Geometry check sheet. Reference: the model listing, model coordinates, mm. Face numbers are marked on the shaded views. A direction names the side the tool comes from. Give positions to 0.01 mm unless a question says otherwise; leave off trailing zeros. Write each loop counter-clockwise with the first axis right and the second up, starting at its lowest first coordinate (ties: lowest second). Pieces come first, ordered by that corner, then holes.
(1) Thickness scan on line 1 along Z through (x, y) = (-20, 0.6); line 2 along X through (y, z) = (13.5, -7.5); line 3 along Z through (x, y) = (-38, 1.6). Record the ranges inside material, lowest first.
(2) Cross-section at A-A (x = -31). Record the boundary of the cut face in (y, z).
(3) Depth check by flat-ended pin: P1, Ø13.5, axis at x = 20, z = 0, coming from the +Y side; P2, Ø0.8, axis at x = 20.5, z = 14.5, coming from the +Y side. Enter the tip coordinate at first touch or a pass-through.
(4) Cross-section at D-D (y = 4). Record the boundary of the cut face in (x, z).
(5) Tool access check on the marked faces 5 and 6. Record the directions out of +Z, -Z, +X, -X, +Y, -Y that give a thin tool (end or side, any length) a straight path to the whole face; none if there is none.
(6) Cross-section at B-B (y = 15.5). Record the boundary of the cut face in (x, z), and give its area (3 significant figures).
(7) Mould release check, pull along Z, two halves, no side actions. Record for the marked faces 1, 2, 3 and 4: +Z half, -Z half, draft (parallel to the pull), parting line (faces both ways), or undercut.
(8) Cross-section at C-C (x = 20). Record the boundary of the cut face in (y, z).
```python
from build123d import *

# Parameters (mm, degrees)
SKETCH2_W              = 105
SKETCH2_H              = 32
BOSS_EXTRUDE1_DEPTH    = 40
SKETCH3_W              = 100
SKETCH3_H              = 32
CUT_EXTRUDE1_DEPTH     = 30
SKETCH4_W              = 100
SKETCH4_H              = 27
CUT_EXTRUDE2_DEPTH     = 7.5
F_10_0MM_DOWEL_HOLE1_D = 10.2
F_2_5MM_DOWEL_HOLE1_D  = 2.6
CIRPATTERN1_COUNT      = 8
F_2_5MM_DOWEL_HOLE2_D  = 2.6
LPATTERN1_COUNT        = 3
LPATTERN1_PITCH        = 38
MIRROR1_COPY_1_D       = 2.6
MIRROR1_COPY_2_D       = 2.6
MIRROR1_COPY_3_D       = 2.6
MIRROR1_COPY_4_D       = 2.6
MIRROR1_COPY_5_D       = 2.6
MIRROR1_COPY_6_D       = 2.6
MIRROR1_COPY_7_D       = 2.6
CUT_EXTRUDE3_DEPTH     = 72.75
F_2_5MM_DOWEL_HOLE3_D  = 2.6
CIRPATTERN3_COUNT      = 5
CIRPATTERN3_ANGLE      = 180
SKETCH18_W             = 16
SKETCH18_H             = 4
CUT_EXTRUDE4_DEPTH     = 72.75
SKETCH19_W             = 10
SKETCH19_H             = 10
SKETCH19_W_2           = 4.5
CUT_EXTRUDE5_DEPTH     = 145.5


with BuildPart() as part:
    # Sketch2 → Boss-Extrude1 (new body)
    with BuildSketch(Plane(origin=(0, 0, 0), x_dir=(1, 0, 0), z_dir=(0, 1, 0))):
        Rectangle(SKETCH2_W, SKETCH2_H)
    extrude(amount=BOSS_EXTRUDE1_DEPTH)

    # Sketch3 → Cut-Extrude1 (cut)
    with BuildSketch(Plane(origin=(0, 40, 0), x_dir=(1, 0, 0), z_dir=(0, 1, 0))):
        Rectangle(SKETCH3_W, SKETCH3_H)
    extrude(amount=-CUT_EXTRUDE1_DEPTH, mode=Mode.SUBTRACT)

    # Sketch4 → Cut-Extrude2 (cut)
    with BuildSketch(Plane(origin=(0, 10, 0), x_dir=(1, 0, 0), z_dir=(0, 1, 0))):
        Rectangle(SKETCH4_W, SKETCH4_H)
    extrude(amount=-CUT_EXTRUDE2_DEPTH, mode=Mode.SUBTRACT)

    # 10.0mm Dowel Hole1 (through all)
    with Locations(Plane(origin=(0, 0, 0), x_dir=(-1, 0, 0), z_dir=(0, -1, 0))):
        with Locations((-20, 0), (20, 0)):
            Hole(F_10_0MM_DOWEL_HOLE1_D / 2)

    # 2.5mm Dowel Hole1 (through all)
    with Locations(Plane(origin=(0, 0, 0), x_dir=(-1, 0, 0), z_dir=(0, -1, 0))):
        with Locations((-20, 11)):
            f_2_5mm_dowel_hole1 = Hole(F_2_5MM_DOWEL_HOLE1_D / 2)

    # CirPattern1: 2.5mm Dowel Hole1 ×8 about axis
    cirpattern1_axis = Axis((20, 0, 0), (0, 1, 0))
    for i in range(1, CIRPATTERN1_COUNT):
        add(f_2_5mm_dowel_hole1.rotate(cirpattern1_axis, i * 360 / CIRPATTERN1_COUNT), mode=Mode.SUBTRACT)

    # 2.5mm Dowel Hole2 (through all)
    with Locations(Plane(origin=(0, 0, 0), x_dir=(-1, 0, 0), z_dir=(0, -1, 0))):
        with Locations((-38, 11), (-38, -11)):
            f_2_5mm_dowel_hole2 = Hole(F_2_5MM_DOWEL_HOLE2_D / 2)

    # LPattern1: 2.5mm Dowel Hole2 ×3
    with Locations(*[(-i * LPATTERN1_PITCH, 0, 0) for i in range(1, LPATTERN1_COUNT)]):
        add(f_2_5mm_dowel_hole2, mode=Mode.SUBTRACT)

    # Mirror1: 2.5mm Dowel Hole1 across plane
    add(f_2_5mm_dowel_hole1.mirror(Plane(origin=(0, 0, 0), x_dir=(0, 0, 1), z_dir=(1, 0, 0))), mode=Mode.SUBTRACT)

    # Mirror1 copy 1 (through all)
    with Locations(Plane(origin=(-5.857864376, 0, 14.142135624), x_dir=(0.707106781, 0, 0.707106781), z_dir=(0, -1, 0))):
        with Locations((-20, -11)):
            Hole(MIRROR1_COPY_1_D / 2)

    # Mirror1 copy 2 (through all)
    with Locations(Plane(origin=(-20, 0, 20), x_dir=(0, 0, 1), z_dir=(0, -1, 0))):
        with Locations((-20, -11)):
            Hole(MIRROR1_COPY_2_D / 2)

    # Mirror1 copy 3 (through all)
    with Locations(Plane(origin=(-34.142135624, 0, 14.142135624), x_dir=(-0.707106781, 0, 0.707106781), z_dir=(0, -1, 0))):
        with Locations((-20, -11)):
            Hole(MIRROR1_COPY_3_D / 2)

    # Mirror1 copy 4 (through all)
    with Locations(Plane(origin=(-40, 0, 0), x_dir=(-1, 0, 0), z_dir=(0, -1, 0))):
        with Locations((-20, -11)):
            Hole(MIRROR1_COPY_4_D / 2)

    # Mirror1 copy 5 (through all)
    with Locations(Plane(origin=(-34.142135624, 0, -14.142135624), x_dir=(-0.707106781, 0, -0.707106781), z_dir=(0, -1, 0))):
        with Locations((-20, -11)):
            Hole(MIRROR1_COPY_5_D / 2)

    # Mirror1 copy 6 (through all)
    with Locations(Plane(origin=(-20, 0, -20), x_dir=(0, 0, -1), z_dir=(0, -1, 0))):
        with Locations((-20, -11)):
            Hole(MIRROR1_COPY_6_D / 2)

    # Mirror1 copy 7 (through all)
    with Locations(Plane(origin=(-5.857864376, 0, -14.142135624), x_dir=(0.707106781, 0, -0.707106781), z_dir=(0, -1, 0))):
        with Locations((-20, -11)):
            Hole(MIRROR1_COPY_7_D / 2)

    # Sketch14 → Cut-Extrude3 (cut, symmetric)
    with BuildSketch(Plane(origin=(0, 0, 0), x_dir=(0, 0, -1), z_dir=(1, 0, 0))):
        with BuildLine():
            Line((-5.1, 40), (5.1, 40))
            Line((5.1, 40), (5.1, 37))
            ThreePointArc((5.1, 37), (0, 31.9), (-5.1, 37))
            Line((-5.1, 37), (-5.1, 40))
        make_face()
    extrude(amount=CUT_EXTRUDE3_DEPTH, both=True, mode=Mode.SUBTRACT)

    # 2.5mm Dowel Hole3 (through all)
    with Locations(Plane(origin=(52.5, 0, 0), x_dir=(0, 0, -1), z_dir=(1, 0, 0))):
        with Locations((11, 37)):
            f_2_5mm_dowel_hole3 = Hole(F_2_5MM_DOWEL_HOLE3_D / 2)

    # CirPattern3: 2.5mm Dowel Hole3 ×5 about axis
    cirpattern3_axis = Axis((0, 37, 0), (-1, 0, 0))
    for i in range(1, CIRPATTERN3_COUNT):
        add(f_2_5mm_dowel_hole3.rotate(cirpattern3_axis, i * CIRPATTERN3_ANGLE / (CIRPATTERN3_COUNT - 1)), mode=Mode.SUBTRACT)

    # Sketch18 → Cut-Extrude4 (cut, symmetric)
    with BuildSketch(Plane(origin=(0, 0, 0), x_dir=(0, 0, -1), z_dir=(1, 0, 0))):
        with Locations((0, 16.5)):
            Rectangle(SKETCH18_W, SKETCH18_H)
        with Locations((0, 8.5)):
            Rectangle(SKETCH18_W, SKETCH18_H)
    extrude(amount=CUT_EXTRUDE4_DEPTH, both=True, mode=Mode.SUBTRACT)

    # Sketch19 → Cut-Extrude5 (cut)
    with BuildSketch(Plane.XZ):
        Rectangle(SKETCH19_W, SKETCH19_H)
        with Locations((40.5, 0)):
            Rectangle(SKETCH19_W_2, SKETCH19_H)
        with Locations((-40.5, 0)):
            Rectangle(SKETCH19_W_2, SKETCH19_H)
    extrude(amount=-CUT_EXTRUDE5_DEPTH, mode=Mode.SUBTRACT)


solid = part.part
```
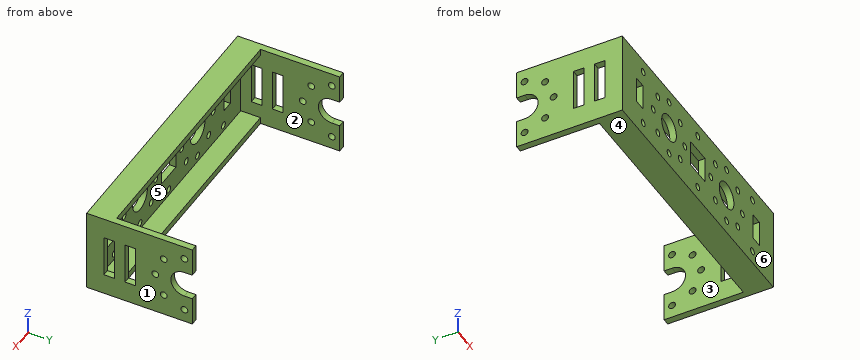
Reply:
1. line 1: z = -16 to -12.3, -9.7 to -5.1, 5.1 to 9.7, 12.3 to 16
1. line 2: x = -52.5 to -50, 50 to 52.5
1. line 3: z = -16 to -12.3, -9.7 to 9.7, 12.3 to 16
2. outline: (0, -16) - (10, -16) - (10, -13.5) - (2.5, -13.5) - (2.5, -1.3) - (0, -1.3) - close; (0, 1.3) - (2.5, 1.3) - (2.5, 13.5) - (10, 13.5) - (10, 16) - (0, 16) - close
3. P1: stops at y = 2.5
3. P2: stops at y = 10
4. outline: (-52.5, -16) - (52.5, -16) - (52.5, 16) - (-52.5, 16) - close; hole (-50, -13.5) - (50, -13.5) - (50, 13.5) - (-50, 13.5) - close
5. face 5: +Y
5. face 6: +Z, -Z, +X, -X, -Y
6. outline: (-52.5, -16) - (-50, -16) - (-50, -8) - (-52.5, -8) - close; (-52.5, 8) - (-50, 8) - (-50, 16) - (-52.5, 16) - close; (50, -16) - (52.5, -16) - (52.5, -8) - (50, -8) - close; (50, 8) - (52.5, 8) - (52.5, 16) - (50, 16) - close
6. area: 80.0 mm2
7. face 1: draft
7. face 2: undercut
7. face 3: undercut
7. face 4: -Z half
8. outline: (0, -16) - (10, -16) - (10, -13.5) - (2.5, -13.5) - (2.5, -12.3) - (0, -12.3) - close; (0, -9.7) - (2.5, -9.7) - (2.5, -5.1) - (0, -5.1) - close; (0, 5.1) - (2.5, 5.1) - (2.5, 9.7) - (0, 9.7) - close; (0, 12.3) - (2.5, 12.3) - (2.5, 13.5) - (10, 13.5) - (10, 16) - (0, 16) - close
